Check sheet for the modelled part. Datum: model origin and axes. Units: mm. Coordinates: 2 decimals unless noted, no trailing zeros. Use a Markdown table: item, result. Add a question column.
1) Go/stop test with flat-tipped pins: P1, Ø0.8, axis at y = 0, z = 456, coming from the +X side; P2, Ø3, axis at y = 1, z = 201.5, coming from the +X side. Record where each tip stops, or that it passes through.
2) Thickness scan on line 1 (Y direction, x = -3, z = -362.5); line 2 (X direction, y = 9, z = -582.5); line 3 (Y direction, x = 4.25, z = -359) (3 decimals). Record the ranges inside material, lowest first.
3) Sectioned sample at A-A, the plane z = 798.5. State how many separate pieces and enclosed holes the cut face has, then the cut area to 3 significant figures.
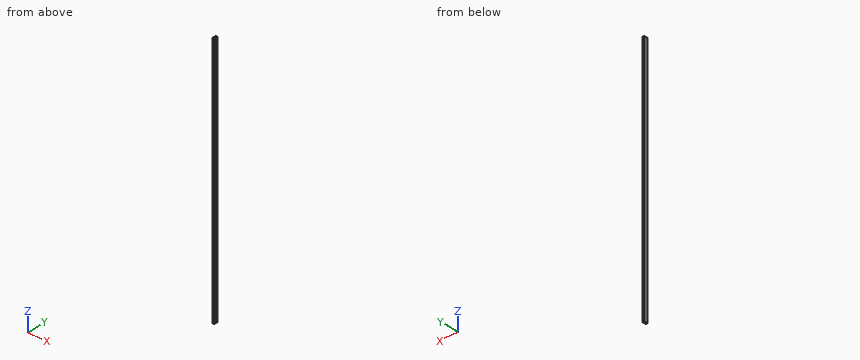
from build123d import *

# Parameters (mm, degrees)
SKETCH3_R           = 2.201333333
SKETCH3_R_2         = 1.693333333
BOSS_EXTRUDE1_DEPTH = 914.4


with BuildPart() as part:
    # Sketch3 → Boss-Extrude1 (new, symmetric)
    with BuildSketch(Plane.XY):
        with BuildLine():
            Line((-1.778, 0), (-1.778, 1.27))
            ThreePointArc((-1.778, 1.27), (-1.536070654, 2.494011801), (-0.846666667, 3.533942971))
            Line((-0.846666667, 3.533942971), (2.413267273, 6.793876912))
            ThreePointArc((2.413267273, 6.793876912), (2.578074335, 6.903997469), (2.772477518, 6.942666667))
            Line((2.772477518, 6.942666667), (3.048, 6.942666667))
            ThreePointArc((3.048, 6.942666667), (3.467078619, 6.769078619), (3.640666667, 6.35))
            Line((3.640666667, 6.35), (3.640666667, 4.301066667))
            ThreePointArc((3.640666667, 4.301066667), (3.948165494, 3.558698827), (4.690533333, 3.2512))
            Line((4.690533333, 3.2512), (5.300133333, 3.2512))
            ThreePointArc((5.300133333, 3.2512), (6.042501173, 3.558698827), (6.35, 4.301066667))
            Line((6.35, 4.301066667), (6.35, 10.583333333))
            ThreePointArc((6.35, 10.583333333), (5.730042687, 12.080042687), (4.233333333, 12.7))
            Line((4.233333333, 12.7), (-4.233333333, 12.7))
            ThreePointArc((-4.233333333, 12.7), (-5.730042687, 12.080042687), (-6.35, 10.583333333))
            Line((-6.35, 10.583333333), (-6.35, 0))
            Line((-6.35, 0), (-1.778, 0))
        make_face()
        with Locations(Location((-2.116666667, 8.466666667, 0), (0, 0, 180))):
            Circle(SKETCH3_R, mode=Mode.SUBTRACT)
        with Locations(Location((3.429, 9.906, 0), (0, 0, 180))):
            Circle(SKETCH3_R_2, mode=Mode.SUBTRACT)
    extrude(amount=BOSS_EXTRUDE1_DEPTH, both=True)

    # Mirror1: part across plane


with BuildPart() as part_1:
    add(part.part)
    add(part.part.mirror(Plane.ZX))


solid = part_1.part
Solved:
| question | item | result |
|---|---|---|
| 1 | P1 | stops at x = -1.78 |
| 1 | P2 | stops at x = -1.53 |
| 2 | line 1 | y = -12.7 to -10.48, -6.45 to 6.45, 10.48 to 12.7 |
| 2 | line 2 | x = -6.35 to -4.25, 0.02 to 2, 4.86 to 6.35 |
| 2 | line 3 | y = -12.7 to -11.387, -8.425 to -3.348, 3.348 to 8.425, 11.387 to 12.7 |
| 3 | separate pieces | 1 |
| 3 | enclosed holes | 4 |
| 3 | area | 196 mm2 |
